from build123d import *

# Parameters (mm, degrees)
SKETCH_1_W                      = 30
SKETCH_1_H                      = 30
EXTRUDE_1_DEPTH                 = 30
CHAMFER_6_SIZE                  = 1
EXTRUDE_3_DEPTH                 = 40
PATTERN_CIRCULAR_8_COUNT        = 2
PATTERN_CIRCULAR_8_ANGLE        = 270
PATTERN_CIRCULAR_8_COPY_1_DEPTH = 40
SKETCH_16_W                     = 12.549729198
SKETCH_16_H                     = 35.597789554
CUT_EXTRUDE_8_DEPTH             = 50
SKETCH_17_W                     = 46.119781587
SKETCH_17_H                     = 25.089994046
CUT_EXTRUDE_10_DEPTH            = 50
CUT_EXTRUDE_2_DEPTH             = 30
PATTERN_CIRCULAR_1_COUNT        = 2
PATTERN_CIRCULAR_1_ANGLE        = 270
PATTERN_CIRCULAR_1_COPY_1_DEPTH = 30
CHAMFER_5_SIZE                  = 1
SKETCH_2_W                      = 26
SKETCH_2_H                      = 26
CUT_EXTRUDE_1_DEPTH             = 28
FILLET_1_R                      = 2
CHAMFER_1_SIZE                  = 1.5
CUT_EXTRUDE_3_DEPTH             = 25
SKETCH_12_W                     = 10
SKETCH_12_H                     = 2
EXTRUDE_6_DEPTH                 = 2
SKETCH_13_R                     = 0.5
CUT_EXTRUDE_6_DEPTH             = 40.446165847
SKETCH_14_W                     = 0.5
SKETCH_14_H                     = 0.5
CUT_EXTRUDE_7_DEPTH             = 1
CHAMFER_8_SIZE                  = 0.5
FILLET_6_R                      = 0.3


with BuildPart() as part:
    # 草图1 → 凸台-拉伸1 (new body)
    with BuildSketch(Plane.XY):
        Rectangle(SKETCH_1_W, SKETCH_1_H)
    extrude(amount=EXTRUDE_1_DEPTH)

    # 倒角6
    chamfer_6_edges = [part.edges().sort_by_distance(p)[0] for p in [
        (-15, 0, 30),
        (0, -15, 30),
        (15, 0, 30),
        (0, 15, 30),
    ]]
    chamfer(chamfer_6_edges, length=CHAMFER_6_SIZE)

    # 草图6 → 凸台-拉伸3 (add)
    with BuildSketch(Plane.XY):
        Polygon((-12.5, 15), (-11.5, 15), (-11.5, 15.8), (-11, 15.8), (-11, 16), (-13, 16), (-13, 15.8), (-12.5, 15.8), align=None)
    extrude_3 = extrude(amount=EXTRUDE_3_DEPTH)

    # 镜向4: 凸台-拉伸3 across plane
    add(extrude_3.mirror(Plane(origin=(0, 0, 0), x_dir=(0, 0, 1), z_dir=(1, 0, 0))))

    # 阵列(圆周)8: 凸台-拉伸3 ×2 about axis
    pattern_circular_8_axis = Axis((0, 0, 0), (0, 0, -1))
    for i in range(1, PATTERN_CIRCULAR_8_COUNT):
        add(extrude_3.rotate(pattern_circular_8_axis, i * PATTERN_CIRCULAR_8_ANGLE / (PATTERN_CIRCULAR_8_COUNT - 1)))

    # 阵列(圆周)8 copy 1 sketch → 阵列(圆周)8 copy 1 (add)
    with BuildSketch(Plane(origin=(0, 0, 0), x_dir=(0, -1, 0), z_dir=(0, 0, 1))):
        Polygon((-12.5, -15), (-11.5, -15), (-11.5, -15.8), (-11, -15.8), (-11, -16), (-13, -16), (-13, -15.8), (-12.5, -15.8), align=None)
    extrude(amount=PATTERN_CIRCULAR_8_COPY_1_DEPTH)

    # 草图16 → 切除-拉伸8 (cut, along a direction that is not the sketch's normal)
    with BuildSketch(Plane(origin=(-22, 0, 22), x_dir=(0.7071067811865475, 0, 0.7071067811865477), z_dir=(-0.7071067811865477, 0, 0.7071067811865475))):
        with Locations((10.913675879, 1.48547553)):
            Rectangle(SKETCH_16_W, SKETCH_16_H)
    extrude(amount=CUT_EXTRUDE_8_DEPTH, dir=(0, 0, 1), mode=Mode.SUBTRACT)

    # 草图17 → 切除-拉伸10 (cut, along a direction that is not the sketch's normal)
    with BuildSketch(Plane(origin=(0, 22, 22), x_dir=(1, 0, 0), z_dir=(0, 0.7071067811865477, 0.7071067811865475))):
        with Locations((-2.061617887, -8.781830855)):
            Rectangle(SKETCH_17_W, SKETCH_17_H)
    extrude(amount=CUT_EXTRUDE_10_DEPTH, dir=(0, 0, 1), mode=Mode.SUBTRACT)

    # 草图8 → 切除-拉伸2 (cut)
    with BuildSketch(Plane.XY.offset(30)):
        Polygon((-12.9, -15), (-11.1, -15), (-11.1, -14.7), (-10.75, -14.7), (-10.75, -13.7), (-13.25, -13.7), (-13.25, -14.7), (-12.9, -14.7), align=None)
    cut_extrude_2 = extrude(amount=-CUT_EXTRUDE_2_DEPTH, mode=Mode.SUBTRACT)

    # 镜向1: 切除-拉伸2 across plane
    add(cut_extrude_2.mirror(Plane(origin=(0, 0, 0), x_dir=(0, 0, 1), z_dir=(1, 0, 0))), mode=Mode.SUBTRACT)

    # 阵列(圆周)1: 切除-拉伸2 ×2 about axis
    pattern_circular_1_axis = Axis((0, 0, 0), (0, 0, -1))
    for i in range(1, PATTERN_CIRCULAR_1_COUNT):
        add(cut_extrude_2.rotate(pattern_circular_1_axis, i * PATTERN_CIRCULAR_1_ANGLE / (PATTERN_CIRCULAR_1_COUNT - 1)), mode=Mode.SUBTRACT)

    # 阵列(圆周)1 copy 1 sketch → 阵列(圆周)1 copy 1 (cut)
    with BuildSketch(Plane(origin=(0, 0, 30), x_dir=(0, -1, 0), z_dir=(0, 0, 1))):
        Polygon((-12.9, 15), (-11.1, 15), (-11.1, 14.7), (-10.75, 14.7), (-10.75, 13.7), (-13.25, 13.7), (-13.25, 14.7), (-12.9, 14.7), align=None)
    extrude(amount=-PATTERN_CIRCULAR_1_COPY_1_DEPTH, mode=Mode.SUBTRACT)

    # 倒角5
    chamfer_5_edges = [part.edges().sort_by_distance(p)[0] for p in [
        (15, -15, 14.5),
        (-15, -15, 14.5),
        (15, 15, 14.5),
        (-15, 15, 14.5),
    ]]
    chamfer(chamfer_5_edges, length=CHAMFER_5_SIZE)

    # 草图2 → 切除-拉伸1 (cut)
    with BuildSketch(Plane(origin=(0, 0, 0), x_dir=(-1, 0, 0), z_dir=(0, 0, -1))):
        Rectangle(SKETCH_2_W, SKETCH_2_H)
    extrude(amount=-CUT_EXTRUDE_1_DEPTH, mode=Mode.SUBTRACT)

    # 圆角1
    fillet_1_edges = [part.edges().sort_by_distance(p)[0] for p in [
        (13, -13, 14),
        (-13, -13, 14),
    ]]
    fillet(fillet_1_edges, radius=FILLET_1_R)

    # 倒角1
    chamfer_1_edges = [part.edges().sort_by_distance(p)[0] for p in [
        (13, 13, 14),
        (-13, 13, 14),
    ]]
    chamfer(chamfer_1_edges, length=CHAMFER_1_SIZE)

    # 草图9 → 切除-拉伸3 (cut)
    with BuildSketch(Plane(origin=(0, 0, 0), x_dir=(-1, 0, 0), z_dir=(0, 0, -1))):
        with BuildLine():
            Line((12.397056275, 14.2), (13.8, 14.2))
            ThreePointArc((13.8, 14.2), (14.082842712, 14.082842712), (14.2, 13.8))
            Line((14.2, 13.8), (14.2, 12.397056275))
            ThreePointArc((14.2, 12.397056275), (13.953073373, 12.027504462), (13.517157288, 12.114213562))
            Line((13.517157288, 12.114213562), (12.114213562, 13.517157288))
            ThreePointArc((12.114213562, 13.517157288), (12.027504462, 13.953073373), (12.397056275, 14.2))
        make_face()
    extrude(amount=-CUT_EXTRUDE_3_DEPTH, mode=Mode.SUBTRACT)

    # 草图12 → 凸台-拉伸6 (add)
    with BuildSketch(Plane(origin=(0, 0, 0), x_dir=(-1, 0, 0), z_dir=(0, 0, -1))):
        with Locations((0, -14)):
            Rectangle(SKETCH_12_W, SKETCH_12_H)
    extrude(amount=EXTRUDE_6_DEPTH)

    # 草图13 → 切除-拉伸6 (cut, through all)
    with BuildSketch(Plane.ZY.offset(5)):
        with Locations(Location((-1, -14, 0), (0, 0, 270))):
            Circle(SKETCH_13_R)
    extrude(amount=-CUT_EXTRUDE_6_DEPTH, mode=Mode.SUBTRACT)

    # 草图14 → 切除-拉伸7 (cut)
    with BuildSketch(Plane(origin=(0, 0, -2), x_dir=(-1, 0, 0), z_dir=(0, 0, -1))):
        with Locations((-4.75, -14)):
            Rectangle(SKETCH_14_W, SKETCH_14_H)
        with Locations((4.75, -14)):
            Rectangle(SKETCH_14_W, SKETCH_14_H)
    extrude(amount=-CUT_EXTRUDE_7_DEPTH, mode=Mode.SUBTRACT)

    # 倒角8
    chamfer_8_edges = [part.edges().sort_by_distance(p)[0] for p in [
        (0, -15, -2),
        (0, -13, -2),
    ]]
    chamfer(chamfer_8_edges, length=CHAMFER_8_SIZE)

    # 圆角6
    # the kernel refuses this fillet: 0.3 mm, written as the material it takes off along each edge
    with BuildSketch(Plane(origin=(-4.5, -14.25, -1.433012702), x_dir=(0, -0.8016059252125737, 0.5978527750743438), z_dir=(-1, 0, 0))) as fillet_6_piece_1:
        with BuildLine():
            CenterArc((0.152038547, -0.297941245), FILLET_6_R, 96.716268279, 46.567463442)
            Line((-0.088443231, -0.118585412), (-0.093252866, -0.114998296))
            Line((-0.093252866, -0.114998296), (-0.004809636, 0.003587117))
            Line((-0.004809636, 0.003587117), (0.000701716, 0.005958825))
            ThreePointArc((0.000701716, 0.005958825), (0.058476364, 0.002568741), (0.116251012, 0.005958825))
            Line((0.116251012, 0.005958825), (0.116952728, 0))
        make_face()
    extrude(amount=0.869837, mode=Mode.SUBTRACT)
    with BuildSketch(Plane(origin=(-4.5, -13.75, -1.433012702), x_dir=(0, 0.8016059252125791, 0.5978527750743364), z_dir=(-1, 0, 0)), Plane(origin=(5.369837, -13.75, -1.433012702), x_dir=(0, 0.8016059252125827, 0.5978527750743317), z_dir=(-1, 0, 0))) as fillet_6_piece_2:
        with BuildLine():
            CenterArc((0.152038547, 0.297941245), FILLET_6_R, 216.716268279, 46.567463442)
            Line((-0.088443231, 0.118585412), (-0.093252866, 0.114998296))
            Line((-0.093252866, 0.114998296), (-0.004809636, -0.003587117))
            Line((-0.004809636, -0.003587117), (0.000701716, -0.005958825))
            ThreePointArc((0.000701716, -0.005958825), (0.058476364, -0.002568741), (0.116251012, -0.005958825))
            Line((0.116251012, -0.005958825), (0.116952728, 0))
        make_face()
    extrude(amount=0.869837, mode=Mode.SUBTRACT)
    with BuildSketch(Plane(origin=(-5.739509973, -14.25, -2), x_dir=(0, -1, 0), z_dir=(1, 0, 0)), Plane(origin=(-4.5, -13.75, -2), x_dir=(0, 1, 0), z_dir=(-1, 0, 0)), Plane(origin=(4.5, -14.25, -2), x_dir=(0, -1, 0), z_dir=(1, 0, 0)), Plane(origin=(5.739509973, -13.75, -2), x_dir=(0, 1, 0), z_dir=(-1, 0, 0))) as fillet_6_piece_3:
        with BuildLine():
            CenterArc((0.3, -0.295803989), FILLET_6_R, 99.594068227, 80.405931773)
            Line((0, -0.295803989), (-0.006, -0.295803989))
            Line((-0.006, -0.295803989), (-0.006, 0))
            Line((-0.006, 0), (0, 0.006))
            ThreePointArc((0, 0.006), (0.125, 0.006), (0.249, 0.00591608))
            Line((0.249, 0.00591608), (0.25, 0))
        make_face()
    extrude(amount=1.239509973, mode=Mode.SUBTRACT)
    with BuildSketch(Plane(origin=(5.369837, -14.25, -1.433012702), x_dir=(0, 0, -1), z_dir=(-1, 0, 0))) as fillet_6_piece_4:
        with BuildLine():
            CenterArc((0.1479348, 0.3), FILLET_6_R, 223.432536558, 46.567463442)
            Line((-0.069920513, 0.09375), (-0.074277619, 0.089625))
            ThreePointArc((-0.074277619, 0.089625), (-0.037019375, 0.045339271), (-0.005196152, -0.003))
            Line((-0.005196152, -0.003), (0, -0.006))
            Line((0, -0.006), (0.1479348, -0.006))
            Line((0.1479348, -0.006), (0.1479348, 0))
        make_face()
    extrude(amount=0.869837, mode=Mode.SUBTRACT)


solid = part.part
Design review of the part built by this model. Coordinates are the model's own, in mm. A direction names the side the tool comes from. Coordinates: 2 decimals unless noted, no trailing zeros. Loops run counter-clockwise (first coordinate to the right, second up) from the corner with the lowest first, then second, coordinate; pieces in that order, holes last.
Item 1: Add section D-D (z = 4). Give the number of separate pieces and of enclosed holes in the cut face, and give its area (3 significant figures).
Completed:
separate pieces: 1
enclosed holes: 2
area: 215 mm2
Item 2: Add section B-B (y = 3.5). Write out the cut boundary in (x, z).
Completed:
outline: (-15, 0) - (-13, 0) - (-13, 28) - (13, 28) - (13, 0) - (15, 0) - (15, 29) - (14, 30) - (-14, 30) - (-15, 29) - close
Item 3: Draft analysis for pull direction Y (two halves, no side actions). For faces 1 (the flat face through (13, 0, 14)), 2 (the flat face through (-0.2, -14.5, 29.5)), 3 (the flat face through (15, 13.4, 14.3)), 4 (the cylindrical face through (-0.07, -13.935, -0.504)), state which applies: pulls with the +Y half, pulls with the -Y half, needs draft (parallel to the pull), parting line crosses it, or undercut.
Completed:
face 1: undercut
face 2: pulls with the -Y half
face 3: needs draft
face 4: undercut
Item 4: Add section A-A (x = -2). Write out the cut boundary in (y, z).
Completed:
outline: (-15, -1.5) - (-14.5, -2) - (-13.5, -2) - (-13, -1.5) - (-13, 28) - (13, 28) - (13, 0) - (15, 0) - (15, 29) - (14, 30) - (-14, 30) - (-15, 29) - close; hole circle Ø1 at (-14, -1)
Item 5: Wall thickness on L1, parallel to X at y = -14, z = 2; L2, parallel to Z at x = 1, y = -14; L3, parallel to X at y = 3, z = 4.5: over which ranges is each line inside the solid? List them lowest first.
Completed:
L1: x = -15 to -13.25, -10.75 to 10.75, 13.25 to 15
L2: z = -2 to -1.5, -0.5 to 30
L3: x = -15 to -13, 13 to 15
Item 6: For faces 5 (the cylindrical face through (-12.4, -12.43, 14.2)), 6 (the flat face through (14, -10.75, 15)), 7 (the flat face through (0, -15, 14)), list the 3-axis set-ups (+Z, -Z, +X, -X, +Y, -Y) from which the entire face can be reached by the end or side of a thin tool; tool diameter is ignored.
Completed:
face 5: -Z
face 6: +Z, -Z
face 7: +Z, -Z, +X, -X, -Y
Item 7: Clearance check with flat-ended pins moving along their axes: pin 1 (1 mm diameter, centred on y = -13.5, z = -1.5, fed in from +X); pin 2 (0.9 mm diameter, centred on x = -15.5, z = 8, fed in from +Y); pin 3 (0.5 mm diameter, centred on x = 14.5, z = 10, fed in from +Y). State where each tip first meets the part, or that it passes through.
Completed:
pin 1: stops at x = 5
pin 2: stops at y = 13
pin 3: stops at y = 14.75
